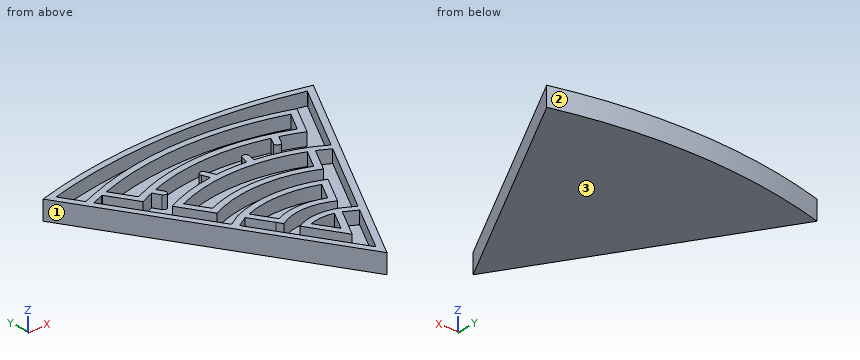
from build123d import *

# Parameters (mm, degrees)
F1_DEPTH = 6
F3_DEPTH = 2


with BuildPart() as f1:
    # F0 (on Top) → F1 (new body)
    with BuildSketch(Plane.XY):
        with BuildLine():
            Line((-43.30127, 25), (0, -50))
            Line((0, -50), (43.30127, 25))
            ThreePointArc((43.30127, 25), (0, 30.847641), (-43.30127, 25))
        make_face()
        with BuildLine():
            ThreePointArc((-11.589333, -13.426687), (-0.072865, -11.565377), (11.378667, -13.79157))
            Line((11.378667, -13.79157), (7.849282, -19.904644))
            ThreePointArc((7.849282, -19.904644), (0.005562, -18.216828), (-7.831448, -19.935535))
            Line((-7.831448, -19.935535), (-11.589333, -13.426687))
        make_face(mode=Mode.SUBTRACT)
        with BuildLine():
            ThreePointArc((-3.730163, -27.039168), (0.060809, -26.321755), (3.894771, -26.754059))
            Line((3.894771, -26.754059), (0, -33.5))
            Line((0, -33.5), (-3.730163, -27.039168))
        make_face(mode=Mode.SUBTRACT)
        with BuildLine():
            Line((9.497942, -29.549082), (0, -46))
            Line((0, -46), (-17.152136, -16.291628))
            Line((-17.152136, -16.291628), (-13.471529, -14.166628))
            Line((-13.471529, -14.166628), (-9.604325, -20.864822))
            Line((-9.604325, -20.864822), (-8.604242, -22.597016))
            ThreePointArc((-8.604242, -22.597016), (0.00573, -20.216832), (8.626059, -22.559227))
            Line((8.626059, -22.559227), (9.626098, -20.82711))
            Line((9.626098, -20.82711), (14.241089, -12.833711))
            Line((14.241089, -12.833711), (14.067922, -12.754568))
            ThreePointArc((14.067922, -12.754568), (-0.045906, -9.565553), (-14.253164, -12.308505))
            Line((-14.253164, -12.308505), (-18.152136, -14.559577))
            Line((-18.152136, -14.559577), (-35.505424, 15.497198))
            Line((-35.505424, 15.497198), (-31.782206, 16.874176))
            Line((-31.782206, 16.874176), (-31.461437, 16.992808))
            Line((-31.461437, 16.992808), (-26.316707, 8.081874))
            ThreePointArc((-26.316707, 8.081874), (-24.126261, 9.085191), (-21.898303, 10.0022))
            Line((-21.898303, 10.0022), (-20.685559, 7.700137))
            ThreePointArc((-20.685559, 7.700137), (-19.334733, 7.281486), (-18.916081, 8.632312))
            Line((-18.916081, 8.632312), (-20.006684, 10.702522))
            ThreePointArc((-20.006684, 10.702522), (-1.149596, 14.176087), (17.863047, 11.691171))
            Line((17.863047, 11.691171), (16.553134, 9.386264))
            ThreePointArc((16.553134, 9.386264), (16.928445, 8.022761), (18.291948, 8.398071))
            Line((18.291948, 8.398071), (19.816809, 11.081198))
            ThreePointArc((19.816809, 11.081198), (23.204445, 9.850646), (26.514425, 8.424332))
            Line((26.514425, 8.424332), (32.475953, 18.75))
            ThreePointArc((32.475953, 18.75), (0, 24.562976), (-32.475953, 18.75))
            Line((-32.475953, 18.75), (-36.519939, 17.25439))
            Line((-36.519939, 17.25439), (-39.837169, 23))
            Line((-39.837169, 23), (-40.264169, 23.739586))
            ThreePointArc((-40.264169, 23.739586), (0, 28.847641), (40.264169, 23.739586))
            Line((40.264169, 23.739586), (39.837169, 23))
            Line((39.837169, 23), (26.334579, -0.387172))
            Line((26.334579, -0.387172), (22.653971, 1.737828))
            Line((22.653971, 1.737828), (22.506193, 1.807767))
            ThreePointArc((22.506193, 1.807767), (15.212654, 4.617264), (7.583376, 6.315231))
            Line((7.583376, 6.315231), (8.163141, 8.512388))
            ThreePointArc((8.163141, 8.512388), (7.451374, 9.734431), (6.229331, 9.022663))
            Line((6.229331, 9.022663), (5.581544, 6.567719))
            ThreePointArc((5.581544, 6.567719), (0.753566, 6.859231), (-4.080781, 6.706128))
            Line((-4.080781, 6.706128), (-4.26912, 7.198283))
            Line((-4.26912, 7.198283), (-5.12863, 9.522317))
            ThreePointArc((-5.12863, 9.522317), (-6.413415, 10.113356), (-7.004454, 8.828571))
            Line((-7.004454, 8.828571), (-6.144944, 6.504537))
            ThreePointArc((-6.144944, 6.504537), (-14.516777, 4.82223), (-22.506193, 1.807767))
            Line((-22.506193, 1.807767), (-22.647311, 1.726292))
            Line((-22.647311, 1.726292), (-17.019315, -8.021681))
            ThreePointArc((-17.019315, -8.021681), (-0.039752, -4.305799), (16.88873, -8.247861))
            Line((16.88873, -8.247861), (21.653971, 0.005778))
            Line((21.653971, 0.005778), (25.334579, -2.119222))
            Line((25.334579, -2.119222), (10.497942, -27.817031))
            Line((10.497942, -27.817031), (6.817334, -25.692031))
            Line((6.817334, -25.692031), (6.626115, -25.606798))
            ThreePointArc((6.626115, -25.606798), (-0.001194, -24.322681), (-6.517118, -26.087024))
            Line((-6.517118, -26.087024), (-6.571243, -26.118273))
            Line((-6.571243, -26.118273), (0, -37.5))
            Line((0, -37.5), (5.817334, -27.424082))
            Line((5.817334, -27.424082), (9.497942, -29.549082))
        make_face(mode=Mode.SUBTRACT)
        with BuildLine():
            ThreePointArc((-19.816809, 0.823719), (0, 4.864628), (19.816809, 0.823719))
            Line((19.816809, 0.823719), (16.065514, -5.673714))
            ThreePointArc((16.065514, -5.673714), (-0.03855, -2.305764), (-16.18426, -5.46804))
            Line((-16.18426, -5.46804), (-19.816809, 0.823719))
        make_face(mode=Mode.SUBTRACT)
        with BuildLine():
            Line((29.542751, 17.669546), (25.685216, 10.988099))
            ThreePointArc((25.685216, 10.988099), (0.059225, 16.195833), (-25.499161, 10.665842))
            Line((-25.499161, 10.665842), (-29.542751, 17.669546))
            ThreePointArc((-29.542751, 17.669546), (0, 22.562976), (29.542751, 17.669546))
        make_face(mode=Mode.SUBTRACT)
    extrude(amount=F1_DEPTH)

    # F2 (on Top) → F3 (join)
    with BuildSketch(Plane.XY):
        with BuildLine():
            Line((-43.30127, 25), (0, -50))
            Line((0, -50), (43.30127, 25))
            ThreePointArc((43.30127, 25), (0, 30.847641), (-43.30127, 25))
        make_face()
    extrude(amount=F3_DEPTH)


solid = f1.part
Input: part model. Units: mm. Frame: model coordinates. Face numbers are marked on the shaded views. Give positions to 0.01 mm unless a question says otherwise; leave off trailing zeros. Order: outer loops, then holes, each group sorted by start corner. A loop starts at its lowest first (then second) coordinate and runs counter-clockwise, first axis right, second up. Notation, with made-up numbers: (58, 25) -> (78, 25) arc R15 ccw to (78, 53) -> close; hole circle Ø8 at (45.25, 27). An arc over 180 degrees is marked (long way). Use one line per item in the form item = value.
1) Section A-A, the plane x = -24.5. Return loops of the section in (y, z).
Response values:
outline = (-7.56, 0) -> (29, 0) -> (29, 6) -> (26.98, 6) -> (26.98, 2) -> (21.3, 2) -> (21.3, 6) -> (19.23, 6) -> (19.23, 2) -> (11.1, 2) -> (11.1, 6) -> (8.92, 6) -> (8.92, 2) -> (-3.56, 2) -> (-3.56, 6) -> (-7.56, 6) -> close
2) Line query: probe 1 along Y at (x, z) = (-28, 4.5); probe 2 along X at (y, z) = (-20, 4.7); probe 3 along X at (y, z) = (-35.5, 3.75). Output: solid intervals per line, ascending.
Response values:
probe_1 = -1.5 to 2.5, 11 to 15, 18.18 to 20.28, 26.4 to 28.43
probe_2 = -17.32 to -15.01, -10.1 to 10.1, 15.01 to 17.32
probe_3 = -8.37 to -6.06, -1.15 to 1.15, 6.06 to 8.37
3) Section B-B, the plane z = 3. Count the separate pieces of the cut face and the enclosed holes in it, and give its area (3 significant figures).
Response values:
separate_pieces = 1
enclosed_holes = 5
area = 1,220 mm^2
4) First-contact query: pin 1 Ø6 at (x, y) = (2, 18) entering from +Z; pin 2 Ø3 at (x, y) = (-9.5, 0.5) entering from +Z. Flat tips, straight axial feed; report the tip coordinate or a pass-through.
Response values:
pin_1 = 6
pin_2 = 2
5) Section C-C, the plane x = 37.5. Return loops of the section in (y, z), and give its area (3 significant figures).
Response values:
outline = (14.95, 0) -> (26.48, 0) -> (26.48, 6) -> (24.43, 6) -> (24.43, 2) -> (18.95, 2) -> (18.95, 6) -> (14.95, 6) -> close
area = 47.3 mm^2
6) Mould query, pull axis X, two halves, no side actions, for the marked faces 1, 2 and 3. Classes: pulls with the +X half, pulls with the -X half, needs draft (parallel to the pull), parting line crosses it, or undercut.
Response values:
face_1 = pulls with the -X half
face_2 = parting line crosses it
face_3 = needs draft
